The listing builds one solid part. Answer for the finished solid, in the listing's coordinates (mm). Face numbers are marked on the shaded views. A direction names the side the tool comes from. Give positions to 0.01 mm unless a question says otherwise; leave off trailing zeros. Order: outer loops, then holes, each group sorted by start corner. A loop starts at its lowest first (then second) coordinate and runs counter-clockwise, first axis right, second up. Notation, with made-up numbers: (18, -13) - (27, -13) arc R30 ccw to (27, 10) - close; hole circle Ø5 at (75, 29.5). An arc over 180 degrees is marked (long way). Use a Markdown table: item, result. Add a question column.
1) Find section B-B, the plane x = 3.75. Determine the outline of the cut face in (y, z).
2) Find section A-A, the plane x = 0.6. Determine the outline of the cut face in (y, z), plus the area to 3 significant figures.
3) Flat-ended cylindrical pins translate along their axes: pin 1 (2 mm diameter, centred on x = 2.5, z = -1.5, fed in from +Y); pin 2 (1.5 mm diameter, centred on x = 3.5, z = -3, fed in from -Y). Find the tip coordinate at first contact, or state that the pin passes through.
4) For the marked faces 4 and 5, determine the directions among +Z, -Z, +X, -X, +Y, -Y from which every point of the face is accessible in a straight line to the end or side of a thin tool.
5) The mould has two halves that part along Z. Classify the marked faces 1, 2 and 3: released by +Z, released by -Z, zero draft, split by the parting line, or undercut.
6) Straight lines are drawn through the part: line 1 (Z direction, x = 3.2, y = 0); line 2 (Y direction, x = 4.5, z = 0); line 3 (X direction, y = -3.25, z = -1.5). For each, find the intervals that lie inside material, in ascending order.
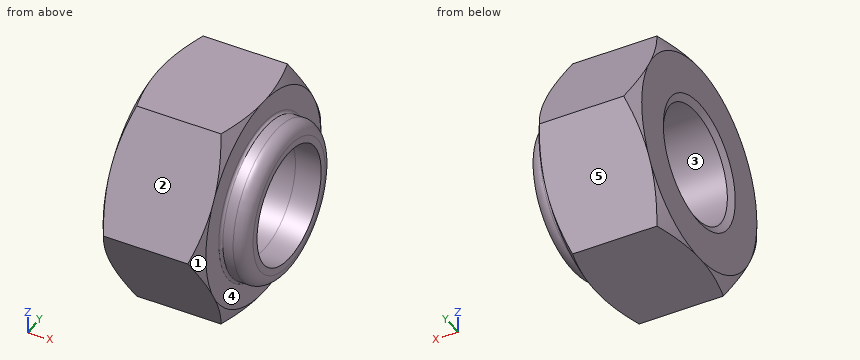
Autodesk Inventor part; units mm, degrees
ref_plane "Work Plane1" through (12.8582, 0, 0) normal (0, 0.8660254, -0.5) x (-1, 0, 0)
ref_plane "Work Plane2" through (2, 0, 0) normal (1, 0, 0) x (0, 0, -1)
ref_plane "YZ Plane" through (0, 0, 0) normal (1, 0, 0) x (0, 1, 0)
sketch "Sketch1" plane through (0, 0, 0) normal (1, 0, 0) x (0, 1, 0)
  line L0 (4.6188, 0) -> (2.3094, -4)
  line L1 (2.3094, -4) -> (-2.3094, -4)
  line L2 (-2.3094, -4) -> (-4.6188, 0)
  line L3 (-4.6188, 0) -> (-2.3094, 4)
  line L4 (-2.3094, 4) -> (2.3094, 4)
  line L5 (2.3094, 4) -> (4.6188, 0)
  point P0 (0, 0)
  point P1 (0, 0)
  dimension "d0" = 9.2376
extrude "Body" add sketch "Sketch1" along normal blind 4
sketch "Sketch2" plane through (0, 0, 0) normal (-1, 0, 0) x (0, 0, 1)
  point P0 (0, 0)
hole "Thread" at (0, 0, 0) direction (1, 0, 0) diameter 4.4587 end through all
chamfer "Chamfer1" distance 0.2706 angle 30 1 edges at (0, 0, -2.2294) measured on face at (0, -2.921, 1.7555)
sketch "Sketch3" plane through (0, 0, 0) normal (0, 0, 1) x (1, 0, 0)
  line L0 (0, 4.6188) -> (4, 4.6188)
  line L1 (4, 2.3094) -> (4, 4.6188)
  line L2 (-0.6, 0) -> (3.6, 0)
  line L3 (3.6427, 4.6188) -> (4, 4)
  dimension "d3" = 8
  dimension "d4" = 30
revolve "Chamfer3" cut sketch "Sketch3" angle 360 about axis through (-10, 0, 0) along (1, 0, 0)
ref_plane "Work Plane1" through (12.8582, 0, 0) normal (0, 0.8660254, -0.5) x (-1, 0, 0)
ref_plane "Work Plane2" through (2, 0, 0) normal (1, 0, 0) x (0, 0, -1)
mirror "Mirror1" about plane through (2, 0, 0) normal (1, 0, 0) of "Chamfer3"
sketch "Sketch6" plane through (4, 0, 0) normal (1, 0, 0) x (0, 0, -1)
  circle A0 centre (0, 0) radius 2.2294
  circle A1 centre (0, 0) radius 3
  dimension "d26" = 6
extrude "Extrusion2" add sketch "Sketch6" along normal blind 1
fillet "Fillet1" radius 0.5 1 edges at (5, 0, 3)
fillet "Fillet2" radius 0.1 1 edges at (4, 0, 3)
equation "\"d13\" = -0.5 * GD1 + 0.5 * NND"
equation "\"d21\" = -0.5 * GD1 + 0.5 * NND"
equation "\"d4\" = ANG2"
equation "\"ANG2\" = 30deg"
equation "\"NND\" = 3"
equation "\"KOH\" = 2.4"
equation "\"SW\" = 5.5"
equation "\"SW01\" = SW"
equation "\"GUL\" = 0.541266 * PTC"
equation "\"TOA\" = 30deg"
equation "\"PTC\" = 0.5"
equation "\"E0\" = 1.155 * SW"
equation "\"THREADDIA\" = 3"
equation "\"GAL\" = 0.541266 * PTC"
properties part number "M3 Nylon Nut" material "Stainless Steel"
The answers:
| question | item | result |
|---|---|---|
| 1 | outline | (-4.42, -0.35) - (-2.51, -3.65) arc R4.43 ccw to (-1.91, -4) - (1.91, -4) arc R4.43 ccw to (2.51, -3.65) - (4.42, -0.35) arc R4.43 ccw to (4.42, 0.35) - (2.51, 3.65) arc R4.43 ccw to (1.91, 4) - (-1.91, 4) arc R4.43 ccw to (-2.51, 3.65) - (-4.42, 0.35) arc R4.43 ccw to start; hole circle Ø4.46 at (0, 0) |
| 2 | outline | (-4.62, 0) - (-2.31, -4) - (2.31, -4) - (4.62, 0) - (2.31, 4) - (-2.31, 4) - close; hole circle Ø4.46 at (0, 0) |
| 2 | area | 39.8 mm2 |
| 3 | pin 1 | y = 4.33 |
| 3 | pin 2 | y = -3.32 |
| 4 | face 4 | +X |
| 4 | face 5 | -Z, +X, -X, +Y |
| 5 | face 1 | split by the parting line |
| 5 | face 2 | released by +Z |
| 5 | face 3 | undercut |
| 6 | line 1 | -4 to -2.23, 2.23 to 4 |
| 6 | line 2 | -3 to -2.23, 2.23 to 3 |
| 6 | line 3 | 0 to 4 |
